Build history of the part. All positions in model axes, mm. A direction names the side the tool comes from. Give positions to 0.01 mm unless a question says otherwise; leave off trailing zeros. One line per item, written item: value. Start each with the question number.
(1) Which spindle directions (+Z, -Z, +X, -X, +Y, -Y) get a long thin tool onto all of the face, cutting with end or side? Do faces 5 (the flat face through (110, -126, -5)), 6 (the flat face through (111.155, -117.274, -8.802)), 7 (the flat face through (99.873, -152.59, 1.937)). Say none if no direction does.
(2) Saw through at A-A on z = -7.5. Count the separate pieces of the cut face and the enclosed holes in it, plus the area to 3 significant figures.
(3) Probe line 1 (Y direction, x = 120, z = -21); line 2 (Z direction, x = 138, y = -117.5); line 3 (Y direction, x = 106.5, z = 6). List the from-to ranges inside material, lowest first.
(4) Two-plate mould, pull along X, no slides. Class faces 1 (the flat face through (103.25, -119.18, 8.2)), 2 (the cylindrical face through (117.8, -135, -18.5)), 3 (the flat face through (111, -128, -12.5)), 4 (the cylindrical face through (105.86, -125.86, -7.03)): +X half, -X half, draft (parallel to the pull), parting line (faces both ways), or undercut.
(5) Pin check, flat tips, straight feed: pin 1 (15 mm diameter, centred on x = 110.5, y = -126, fed in from -Z); pin 2 (3 mm diameter, centred on y = -149, z = -3.5, fed in from +X); pin 3 (5.5 mm diameter, centred on x = 114, y = -125, fed in from +Z). Stop position of each tip, or through.
```python
from build123d import *

# Parameters (mm, degrees)
CYLINDER039_R             = 4.5
CYLINDER039_DEPTH         = 21
ARRAY005_COUNT            = 4
CYLINDER038_R             = 2.5
CYLINDER038_DEPTH         = 21
ARRAY004_COUNT            = 4
FUSION016_PLACEMENT_ANGLE = 90
CYLINDER037_R             = 39
CYLINDER037_DEPTH         = 10
CHAMFER004_SIZE           = 8.4
CYLINDER029_R             = 2.5
CYLINDER029_DEPTH         = 32
CYLINDER028_R             = 4.5
CYLINDER028_DEPTH         = 5
CYLINDER030_R             = 4.5
CYLINDER030_DEPTH         = 5
BOX010_W                  = 24
BOX010_H                  = 14
BOX010_DEPTH              = 10
BOX009_W                  = 18
BOX009_H                  = 10
BOX009_DEPTH              = 21
BOX008_W                  = 21
BOX008_H                  = 22
BOX008_DEPTH              = 24
CHAMFER001_SIZE           = 7
FILLET001_R               = 2
FUSION017_PLACEMENT_ANGLE = 221


with BuildPart() as array005:
    # Cylinder039 → Cylinder039 (new body)
    with BuildSketch(Plane(origin=(23, 0, 0), x_dir=(1, 0, 0), z_dir=(0, 0, 1))):
        Circle(CYLINDER039_R)
    extrude(amount=CYLINDER039_DEPTH)

    # Array005: Array005 ×4 about axis
    array005_axis = Axis((0, 0, 0), (0, 0, 1))


with BuildPart() as array005_1:
    add(array005.part)
    for i in range(1, ARRAY005_COUNT):
        add(array005.part.rotate(array005_axis, i * 360 / ARRAY005_COUNT))


with BuildPart() as array005_2:
    # Array005 placement: moved
    add(array005_1.part.moved(Location((0, 0, -20))))


with BuildPart() as fusion016:
    # Cylinder038 → Cylinder038 (new body)
    with BuildSketch(Plane(origin=(23, 0, 0), x_dir=(1, 0, 0), z_dir=(0, 0, 1))):
        Circle(CYLINDER038_R)
    extrude(amount=CYLINDER038_DEPTH)

    # Array004: Fusion016 ×4 about axis
    array004_axis = Axis((0, 0, 0), (0, 0, 1))


with BuildPart() as fusion016_1:
    add(fusion016.part)
    for i in range(1, ARRAY004_COUNT):
        add(fusion016.part.rotate(array004_axis, i * 360 / ARRAY004_COUNT))

    # Fusion016: union Array005
    add(array005_2.part)


with BuildPart() as fusion016_2:
    # Fusion016 placement: moved
    add(fusion016_1.part.moved(Location((14.5, -61, 0))).rotate(Axis((14.5, -61, 0), (-1, 0, 0)), FUSION016_PLACEMENT_ANGLE))


with BuildPart() as cut034:
    # Cylinder037 → Cylinder037 (new body)
    with BuildSketch(Plane(origin=(14.5, -70, 0), x_dir=(1, 0, 0), z_dir=(0, 1, 0))):
        Circle(CYLINDER037_R)
    extrude(amount=CYLINDER037_DEPTH)

    # Chamfer004
    chamfer004_edges = [cut034.edges().sort_by_distance(p)[0] for p in [
        (-24.5, -70, 0),
    ]]
    chamfer(chamfer004_edges, length=CHAMFER004_SIZE)


with BuildPart() as cut034_1:
    # Chamfer004 placement: moved
    add(cut034.part.moved(Location((0, 7, 0))))

    # Cut034: cut Fusion016
    add(fusion016_2.part, mode=Mode.SUBTRACT)


with BuildPart() as cylinder029:
    # Cylinder029 → Cylinder029 (new body)
    with BuildSketch(Plane(origin=(55, -39, -20), x_dir=(1, 0, 0), z_dir=(0, 0, 1))):
        Circle(CYLINDER029_R)
    extrude(amount=CYLINDER029_DEPTH)


with BuildPart() as cylinder028:
    # Cylinder028 → Cylinder028 (new body)
    with BuildSketch(Plane(origin=(55, -39, 8), x_dir=(1, 0, 0), z_dir=(0, 0, 1))):
        Circle(CYLINDER028_R)
    extrude(amount=CYLINDER028_DEPTH)


with BuildPart() as cylinder030:
    # Cylinder030 → Cylinder030 (new body)
    with BuildSketch(Plane(origin=(55, -39, -14), x_dir=(1, 0, 0), z_dir=(0, 0, 1))):
        Circle(CYLINDER030_R)
    extrude(amount=CYLINDER030_DEPTH)


with BuildPart() as box010:
    # Box010 → Box010 (new body)
    with BuildSketch(Plane(origin=(43, -46, -5), x_dir=(1, 0, 0), z_dir=(0, 0, 1))):
        with Locations((12, 7)):
            Rectangle(BOX010_W, BOX010_H)
    extrude(amount=BOX010_DEPTH)


with BuildPart() as box009:
    # Box009 → Box009 (new body)
    with BuildSketch(Plane(origin=(46, -30, -11), x_dir=(1, 0, 0), z_dir=(0, 0, 1))):
        with Locations((9, 5)):
            Rectangle(BOX009_W, BOX009_H)
    extrude(amount=BOX009_DEPTH)


with BuildPart() as fusion017:
    # Box008 → Box008 (new body)
    with BuildSketch(Plane(origin=(44.5, -45, -12.5), x_dir=(1, 0, 0), z_dir=(0, 0, 1))):
        with Locations((10.5, 11)):
            Rectangle(BOX008_W, BOX008_H)
    extrude(amount=BOX008_DEPTH)

    # Cut025: cut Box009
    add(box009.part, mode=Mode.SUBTRACT)

    # Chamfer001
    chamfer001_edges = [fusion017.edges().sort_by_distance(p)[0] for p in [
        (44.5, -45, -0.5),
        (65.5, -45, -0.5),
    ]]
    chamfer(chamfer001_edges, length=CHAMFER001_SIZE)

    # Fillet001
    fillet001_edges = [fusion017.edges().sort_by_distance(p)[0] for p in [
        (51.5, -45, -0.5),
        (58.5, -45, -0.5),
    ]]
    fillet(fillet001_edges, radius=FILLET001_R)

    # Cut024: cut Box010
    add(box010.part, mode=Mode.SUBTRACT)

    # Cut027: cut Cylinder030
    add(cylinder030.part, mode=Mode.SUBTRACT)

    # Cut026: cut Cylinder028
    add(cylinder028.part, mode=Mode.SUBTRACT)

    # Cut023: cut Cylinder029
    add(cylinder029.part, mode=Mode.SUBTRACT)


with BuildPart() as fusion017_1:
    # Cut023 placement: moved
    add(fusion017.part.moved(Location((-40, -38, 0))))

    # Fusion017: union Cut034
    add(cut034_1.part)


with BuildPart() as fusion017_2:
    # Fusion017 placement: moved
    add(fusion017_1.part.moved(Location((169, -172, 0))).rotate(Axis((169, -172, 0), (0, 0, 1)), FUSION017_PLACEMENT_ANGLE))


solid = fusion017_2.part
```
Results below:
1. face 5: -X, +Y
1. face 6: +Z, -Z, +Y
1. face 7: none
2. separate pieces: 1
2. enclosed holes: 2
2. area: 954 mm²
3. line 1: y = -144.37 to -140.02, -135.45 to -135.09, -131.59 to -131.12
3. line 2: z = -17.63 to -2.31, 2.31 to 17.63
3. line 3: y = -156.1 to -142.85, -138.97 to -136.68, -136.23 to -126.14, -121.32 to -116.96
4. face 1: -X half
4. face 2: undercut
4. face 3: draft
4. face 4: undercut
5. pin 1: stops at z = -12.5
5. pin 2: stops at x = 116.4
5. pin 3: stops at z = 11.5
